Print and shaded views of the part. All mm, measured from the part's lowest x, y and z. A direction names the side the tool comes from. Give positions to 0.01 mm unless a question says otherwise; leave off trailing zeros. Loops run counter-clockwise (first coordinate to the right, second up) from the corner with the lowest first, then second, coordinate; pieces in that order, holes last. Notation, with made-up numbers: M 10,82 L 31,82 A25 ccw 31,97 Z; hole C -36.5,9 d1. An arc over 180 degrees is marked long. Put each result on its own line as item: value. Start each with the question number.
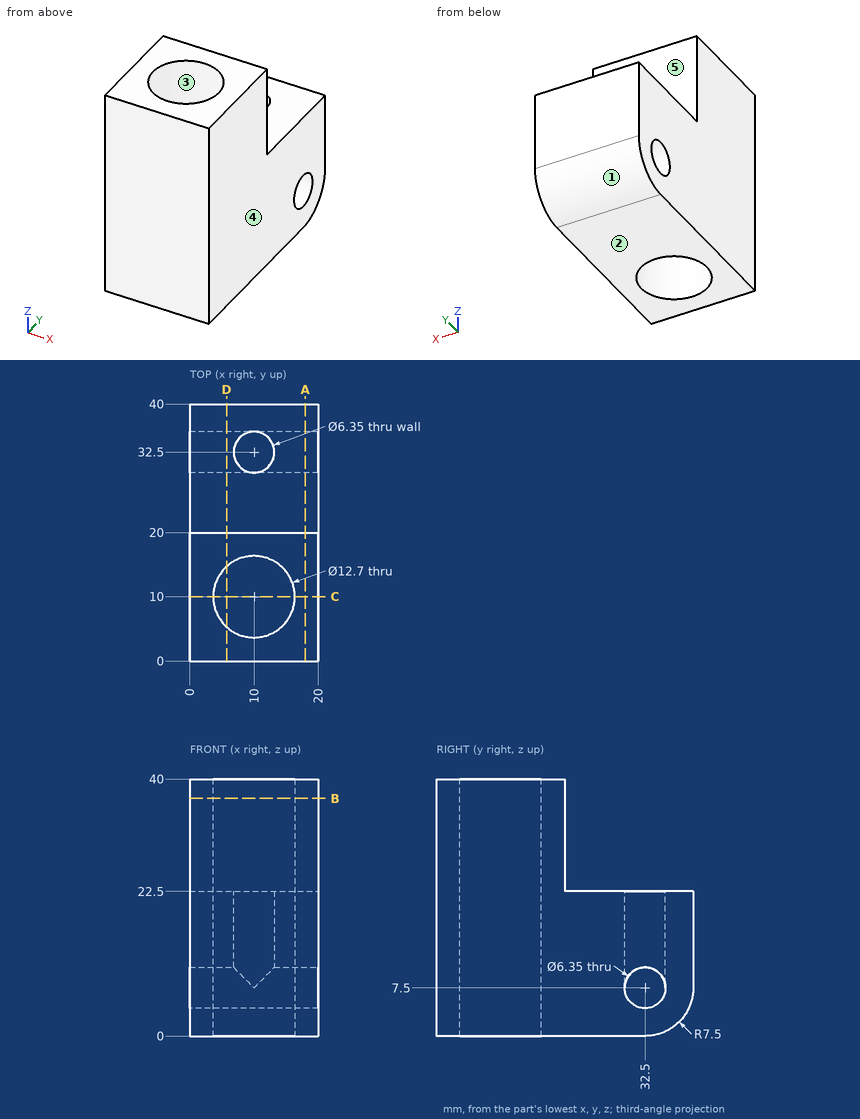
1) Wall check: L1, parallel to Y at x = 10, z = 14.5 (3 decimals); L2, parallel to X at y = 32.5, z = 17.75 (3 decimals); L3, parallel to Y at x = 7.25, z = 20.5. Give the ranges that are in metal, low to high.
2) Band-saw the part on A-A on x = 18. Give the cut face in (y, z) (3 decimals), then the cut area to 3 significant figures.
3) Pin check, flat tips, straight feed: pin 1 Ø4 at (x, y) = (15.5, 28.5) entering from +Z; pin 2 Ø5 at (x, z) = (10, 33.5) entering from +Y. Stop position of each tip, or through.
4) Band-saw the part on B-B on z = 37. Give the cut face in (x, y), then the cut area to 3 significant figures.
5) Band-saw the part on D-D on x = 5.75. Give the cut face in (y, z) (3 decimals).
6) Mould opens along Y. For the marked faces 1, 2 and 3 say: +Y half, -Y half, draft (parallel to the pull), parting line (faces both ways), or undercut.
7) Band-saw the part on C-C on y = 10. Give the cut face in (x, z), then the cut area to 3 significant figures.
8) Which spindle directions (+Z, -Z, +X, -X, +Y, -Y) get a long thin tool onto all of the face, cutting with end or side? Do the marked faces 4 and 5. Say none if no direction does.
Evaluation:
1. L1: 0 to 3.65, 16.35 to 29.325, 35.675 to 40
1. L2: 0 to 6.825, 13.175 to 20
1. L3: 0 to 4.28, 15.72 to 30.91, 34.09 to 40
2. outline: M 0,0 L 32.5,0 A7.5 ccw 40,7.5 L 40,22.5 L 20,22.5 L 20,40 L 0,40 Z; hole C 32.5,7.5 d6.35
2. area: 1,210 mm2
3. pin 1: z = 22.5
3. pin 2: y = 20
4. outline: M 0,0 L 20,0 L 20,20 L 0,20 Z; hole C 10,10 d12.7
4. area: 273 mm2
5. outline: M 0,0 L 5.282,0 L 5.282,40 L 0,40 Z; M 14.718,0 L 32.5,0 A7.5 ccw 40,7.5 L 40,22.5 L 20,22.5 L 20,40 L 14.718,40 Z; hole C 32.5,7.5 d6.35
6. face 1: +Y half
6. face 2: draft
6. face 3: undercut
7. outline: M 0,0 L 3.65,0 L 3.65,40 L 0,40 Z; M 16.35,0 L 20,0 L 20,40 L 16.35,40 Z
7. area: 292 mm2
8. face 4: +Z, -Z, +X, +Y, -Y
8. face 5: +Z, +X, -X, +Y
